Print and shaded views of the part. All mm, measured from the part's lowest x, y and z. A direction names the side the tool comes from. Round coordinates to 2 decimals unless told otherwise and drop trailing zeros. Loops run counter-clockwise (first coordinate to the right, second up) from the corner with the lowest first, then second, coordinate; pieces in that order, holes last. Notation, with made-up numbers: (-21.75, 16.25) -> (-1.75, 16.25) arc R13 ccw to (-1.75, 25.25) -> close; hole circle Ø9 at (25, 29). An arc over 180 degrees is marked (long way). Use a Markdown table: item, result.
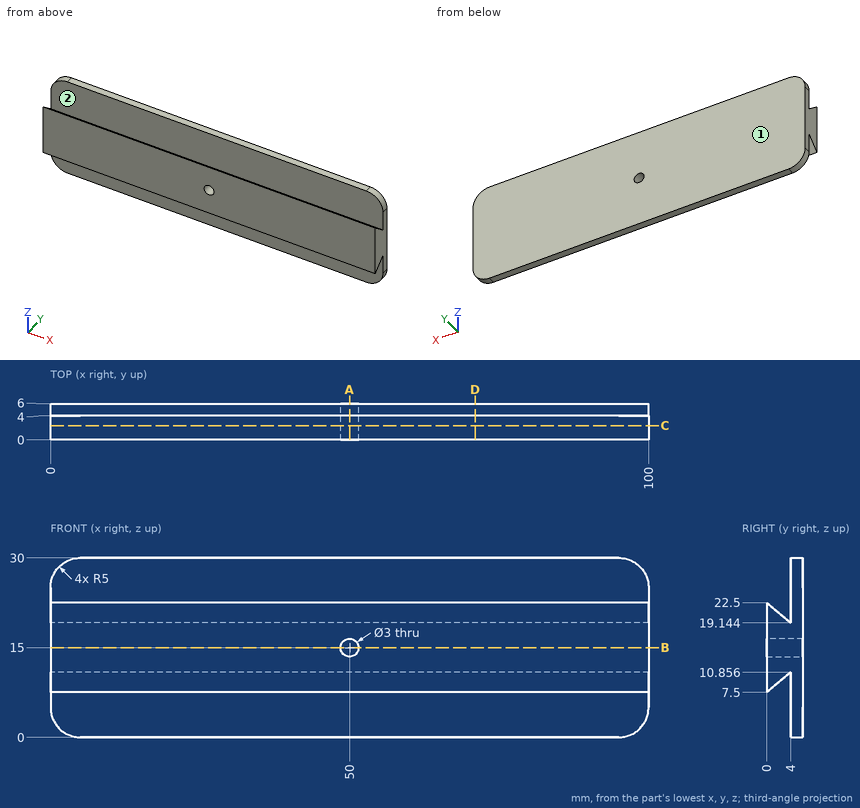
Q1. Flat gauge pin, fed straight in: pin 1 (5.5 mm diameter, centred on x = 61, z = 25.5, fed in from -Y). Where does the tip first touch, or does it go through?
Results list:
| item | result |
|---|---|
| pin 1 | stops at y = 4 |
Q2. Drill centre lines: L1, parallel to X at y = 1.25, z = 15; L2, parallel to Y at x = 12, z = 26; L3, parallel to Y at x = 58, z = 8 (1 decimal). Where is each one in solid material? Low to high. Write a range as from..to.
Results list:
| item | result |
|---|---|
| L1 | x = 0..48.5, 51.5..100 |
| L2 | y = 4..6 |
| L3 | y = 0..0.6, 4..6 |
Q3. Band-saw the part on A-A, the plane x = 50. Give the cut face in (y, z).
Results list:
| item | result |
|---|---|
| outline | (0, 7.5) -> (4, 10.86) -> (4, 0) -> (6, 0) -> (6, 13.5) -> (0, 13.5) -> close; (0, 16.5) -> (6, 16.5) -> (6, 30) -> (4, 30) -> (4, 19.14) -> (0, 22.5) -> close |
Q4. Tool access for the marked faces 1 and 2: list every direction of +Z, -Z, +X, -X, +Y, -Y with a clear straight run to the whole face (end or side of a thin tool).
Results list:
| item | result |
|---|---|
| face 1 | +Z, -Z, +X, -X, +Y |
| face 2 | +Z, +X, -X |
Q5. Band-saw the part on C-C, the plane y = 2.4. Give the cut face in (x, z), plus the area to 3 significant figures.
Results list:
| item | result |
|---|---|
| outline | (0, 9.51) -> (100, 9.51) -> (100, 20.49) -> (0, 20.49) -> close; hole circle Ø3 at (50, 15) |
| area | 1,090 mm² |
Q6. Band-saw the part on B-B, the plane z = 15. Give the cut face in (x, y).
Results list:
| item | result |
|---|---|
| outline | (0, 0) -> (48.5, 0) -> (48.5, 6) -> (0, 6) -> close; (51.5, 0) -> (100, 0) -> (100, 6) -> (51.5, 6) -> close |
Q7. Band-saw the part on D-D, the plane x = 71. Give the cut face in (y, z), plus the area to 3 significant figures.
Results list:
| item | result |
|---|---|
| outline | (0, 7.5) -> (4, 10.86) -> (4, 0) -> (6, 0) -> (6, 30) -> (4, 30) -> (4, 19.14) -> (0, 22.5) -> close |
| area | 107 mm² |
